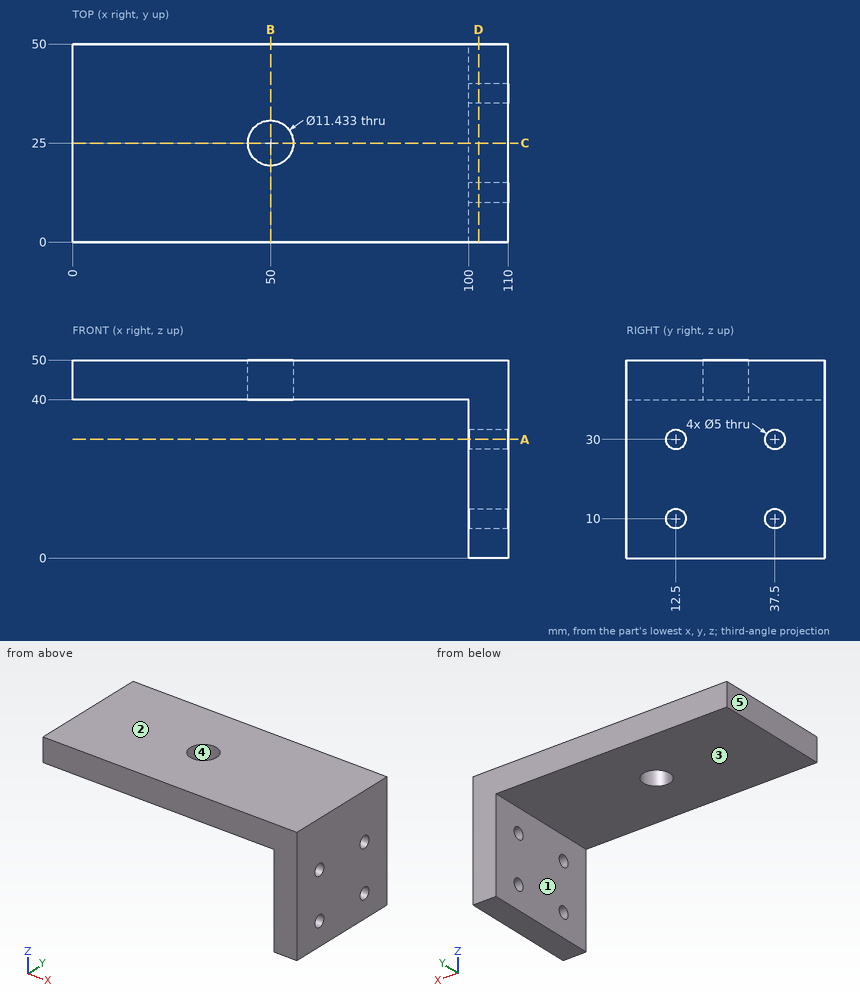
The figure shows three views and two pictorial views of one solid part (mm, origin at its lowest corner). Answer the questions. A direction names the side the tool comes from. Coordinates: 2 decimals unless noted, no trailing zeros. Loops run counter-clockwise (first coordinate to the right, second up) from the corner with the lowest first, then second, coordinate; pieces in that order, holes last. Notation, with made-up numbers: (-26, 76) - (-1, 76) arc R30 ccw to (-1, 104) - close; hole circle Ø8 at (12.25, 31.25). An arc over 180 degrees is marked (long way). Use a Markdown table: item, result. Add a question column.
1) For the marked faces 1 and 2, determine the directions among +Z, -Z, +X, -X, +Y, -Y from which every point of the face is accessible in a straight line to the end or side of a thin tool.
2) The part is cut by section D-D, the plane x = 102.5. Give the vertices of the cut face in (y, z), and give its area (3 significant figures).
3) The part is cut by section A-A, the plane z = 30. Give the vertices of the cut face in (x, y).
4) The part is cut by section C-C, the plane y = 25. Give the vertices of the cut face in (x, z), and give its area (3 significant figures).
5) The part is cut by section B-B, the plane x = 50. Give the vertices of the cut face in (y, z), and give its area (3 significant figures).
6) The mould has two halves that part along X. Classify the marked faces 3, 4 and 5: released by +X, released by -X, zero draft, split by the parting line, or undercut.
7) Find the intervals of material crossed by line 1 (Y direction, x = 107.25, z = 30); line 2 (Y direction, x = 50, z = 46.5); line 3 (Z direction, x = 106, y = 37), in increasing order.
8) Given pin 1 (6.5 mm diameter, centred on y = 12.5, z = 30, fed in from -X); pin 2 (10.5 mm diameter, centred on x = 50, y = 25, fed in from +Z); pin 3 (25 mm diameter, centred on x = 36.5, y = 13, fed in from -Z), each flat-ended and moving along its own axis, determine where each tip first touches the part or whether it passes through.
Here are the results:
| question | item | result |
|---|---|---|
| 1 | face 1 | -Z, -X, +Y, -Y |
| 1 | face 2 | +Z, +X, -X, +Y, -Y |
| 2 | outline | (0, 0) - (50, 0) - (50, 50) - (0, 50) - close; hole circle Ø5 at (12.5, 10); hole circle Ø5 at (12.5, 30); hole circle Ø5 at (37.5, 10); hole circle Ø5 at (37.5, 30) |
| 2 | area | 2,420 mm^2 |
| 3 | outline | (100, 0) - (110, 0) - (110, 10) - (100, 10) - close; (100, 15) - (110, 15) - (110, 35) - (100, 35) - close; (100, 40) - (110, 40) - (110, 50) - (100, 50) - close |
| 4 | outline | (0, 40) - (44.28, 40) - (44.28, 50) - (0, 50) - close; (55.72, 40) - (100, 40) - (100, 0) - (110, 0) - (110, 50) - (55.72, 50) - close |
| 4 | area | 1,390 mm^2 |
| 5 | outline | (0, 40) - (19.28, 40) - (19.28, 50) - (0, 50) - close; (30.72, 40) - (50, 40) - (50, 50) - (30.72, 50) - close |
| 5 | area | 386 mm^2 |
| 6 | face 3 | zero draft |
| 6 | face 4 | undercut |
| 6 | face 5 | released by -X |
| 7 | line 1 | y = 0 to 10, 15 to 35, 40 to 50 |
| 7 | line 2 | y = 0 to 19.28, 30.72 to 50 |
| 7 | line 3 | z = 0 to 7.55, 12.45 to 27.55, 32.45 to 50 |
| 8 | pin 1 | stops at x = 100 |
| 8 | pin 2 | passes through |
| 8 | pin 3 | stops at z = 40 |
